CAD build for the part. Positions are in the model's coordinates, mm. Face numbers are marked on the shaded views. A direction names the side the tool comes from. Coordinates: 2 decimals unless noted, no trailing zeros. Order: outer loops, then holes, each group sorted by start corner. A loop starts at its lowest first (then second) coordinate and runs counter-clockwise, first axis right, second up. Notation, with made-up numbers: (-11.75, 23) - (-6.75, 23) arc R30 ccw to (-6.75, 52) - close; hole circle Ø3 at (43.5, -11). An arc over 180 degrees is marked (long way). Write each question's results on one line, items separated by ' | '. Start each with the question number.
Q1. Pin check, flat tips, straight feed: P1, Ø2.5, axis at y = -3, z = 8, coming from the +X side; P2, Ø5, axis at x = 21.5, z = 3, coming from the +Y side. Stop position of each tip, or through.
Q2. Which spindle directions (+Z, -Z, +X, -X, +Y, -Y) get a long thin tool onto all of the face, cutting with end or side? Do the marked faces 1 and 2. Say none if no direction does.
Q3. Band-saw the part on A-A, the plane x = 16. Write the cut outline in (y, z).
Q4. Wall check: probe 1 along X at (y, z) = (6.25, -4.75); probe 2 along Z at (x, y) = (-1.5, 6.5); probe 3 along Z at (x, y) = (8, -1.5). Give the ranges that are in metal, low to high.
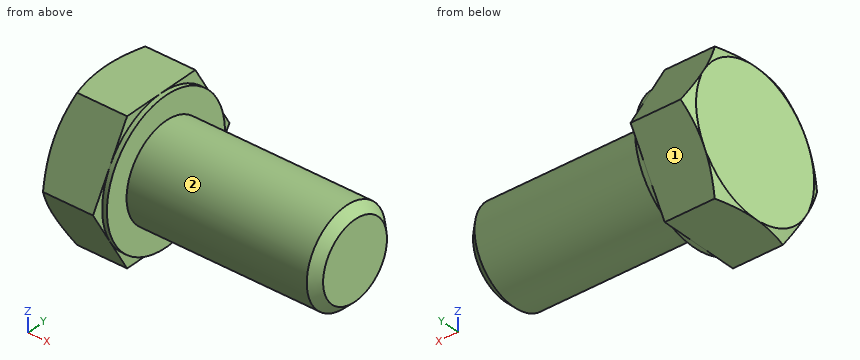
Autodesk Inventor part; units mm, degrees
ref_plane "Work Plane1" through (1.525, 0, 0) normal (0, 0, 1) x (1, 0, 0)
ref_plane "YZ Plane" through (0, 0, 0) normal (1, 0, 0) x (0, 1, 0)
ref_plane "XZ Plane" through (0, 0, 0) normal (0, 1, 0) x (-1, 0, 0)
sketch "Sketch1" plane through (0, 0, 0) normal (0, 0, 1) x (1, 0, 0)
  line L0 (0, 9.525) -> (0, 6.35)
  line L1 (5.969, 6.35) -> (25.4, 6.35)
  line L2 (25.4, 6.35) -> (25.4, 0)
  line L3 (25.4, 0) -> (-0.6351, 0)
  line L4 (-5.8421, 0) -> (30.607, 0)
  line L5 (-0.6351, 0) -> (-0.6351, 9.525)
  line L6 (-0.6351, 9.525) -> (0, 9.525)
  line L7 (5.969, 6.35) -> (0.0024, 6.35)
  line L8 (0.0024, 6.35) -> (0, 6.35)
  line L9 (0, -1.905) -> (0, 11.43)
  dimension "d0" = 25.4
  dimension "d1" = 19.431
  dimension "d2" = 12.7
  dimension "d9" = 0.6351
  dimension "d10" = 19.05
  dimension "d13" = 5.9666
  dimension "d14" = 12.7
revolve "Body" add sketch "Sketch1" angle 360 about axis through (25.4, 0, 0) along (-1, 0, 0)
sketch "Sketch2" plane through (-0.6351, 0, 0) normal (-1, 0, 0) x (0, 0, 1)
  line L0 (0, 10.9985) -> (9.525, 5.4993)
  line L1 (9.525, 5.4993) -> (9.525, -5.4993)
  line L2 (9.525, -5.4993) -> (0, -10.9985)
  line L3 (0, -10.9985) -> (-9.525, -5.4993)
  line L4 (-9.525, -5.4993) -> (-9.525, 5.4993)
  line L5 (-9.525, 5.4993) -> (0, 10.9985)
  point P0 (0, 0)
  point P1 (0, 0)
  dimension "d11" = 19.05
extrude "Head" add sketch "Sketch2" along normal blind 7.5692
sketch "Sketch4" plane through (0, 0, 0) normal (0, 0, 1) x (1, 0, 0)
  line L0 (-8.2043, 9.525) -> (-8.2043, 10.9985)
  line L1 (-8.2043, 10.9985) -> (-7.3536, 10.9985)
  line L2 (-7.3536, 10.9985) -> (-8.2043, 9.525)
  line L3 (-9.7181, 0) -> (0.8787, 0)
  line L4 (-0.6351, 10.9985) -> (-8.2043, 10.9985)
  line L5 (-8.2043, 5.4993) -> (-8.2043, 10.9985)
  dimension "d5" = 30
  dimension "d19" = 19.05
revolve "Chamfer1" cut sketch "Sketch4" angle 360 about axis through (-10, 0, 0) along (1, 0, 0)
thread "Thread"
chamfer "Chamfer2" distance 1.1985 distance2 1.1987 1 edges at (25.4, -6.35, 0) measured on face at (25.4, -1.4034, 0.0866)
ref_plane "Work Plane1" through (1.525, 0, 0) normal (0, 0, 1) x (1, 0, 0)
equation "\"d0\" = NLG"
equation "\"d1\" = GEL"
equation "\"d2\" = GD"
equation "\"d10\" = SD2"
equation "\"d14\" = BDM"
equation "\"d11\" = SW"
equation "\"d3\" = KOH - SD"
equation "\"d5\" = ANG1"
equation "\"d19\" = SW0"
equation "\"d15\" = GEL"
equation "\"d6\" = -0.5 * SPD + 0.5 * GD"
equation "\"NLG\" = 25.4"
equation "\"GD\" = 12.7"
equation "\"BDM\" = 12.7"
equation "\"KOH\" = 8.2042"
equation "\"GEL\" = 19.431"
equation "\"SW\" = 19.05"
equation "\"SW0\" = SW"
equation "\"SPD\" = GD1"
equation "\"SD2\" = SW"
equation "\"SD\" = 0.635"
equation "\"ANG1\" = 30deg"
equation "\"GAL\" = 5.96646"
equation "\"GUL\" = 1.19863"
equation "\"RR\" = 0.381"
equation "\"WFT\" = SD"
equation "\"GD1\" = 10.303"
equation "\"THREADDIA\" = 12.7"
equation "\"SDH\" = SW"
equation "\"SDHG\" = 0.00254"
equation "\"TOA\" = 30deg"
equation "\"FAWI\" = 45deg"
equation "\"NND\" = 12.7"
equation "\"E0\" = 22.00275"
properties part number "AS 2465 - 1/2 x 1  UNC" material "Steel, Mild"
Results below:
1) P1: stops at x = 0 | P2: stops at y = 6.33
2) face 1: -Z, +X, -X, +Y | face 2: +X
3) outline: circle Ø12.7 at (0, 0)
4) probe 1: x = -8.2 to 0 | probe 2: z = -7.79 to 7.79 | probe 3: z = -6.17 to 6.17
